Input: dimensioned drawing with shaded views. Units: mm. Origin: part minimum x, y, z. Round coordinates to 2 decimals unless told otherwise and drop trailing zeros. Loops run counter-clockwise (first coordinate to the right, second up) from the corner with the lowest first, then second, coordinate; pieces in that order, holes last. Notation, with made-up numbers: M -12,36 L -2,36 A24 ccw -2,72 Z; hole C 77,73.5 d5. An arc over 180 degrees is marked long. Answer as a JSON object with one key per item and string values.
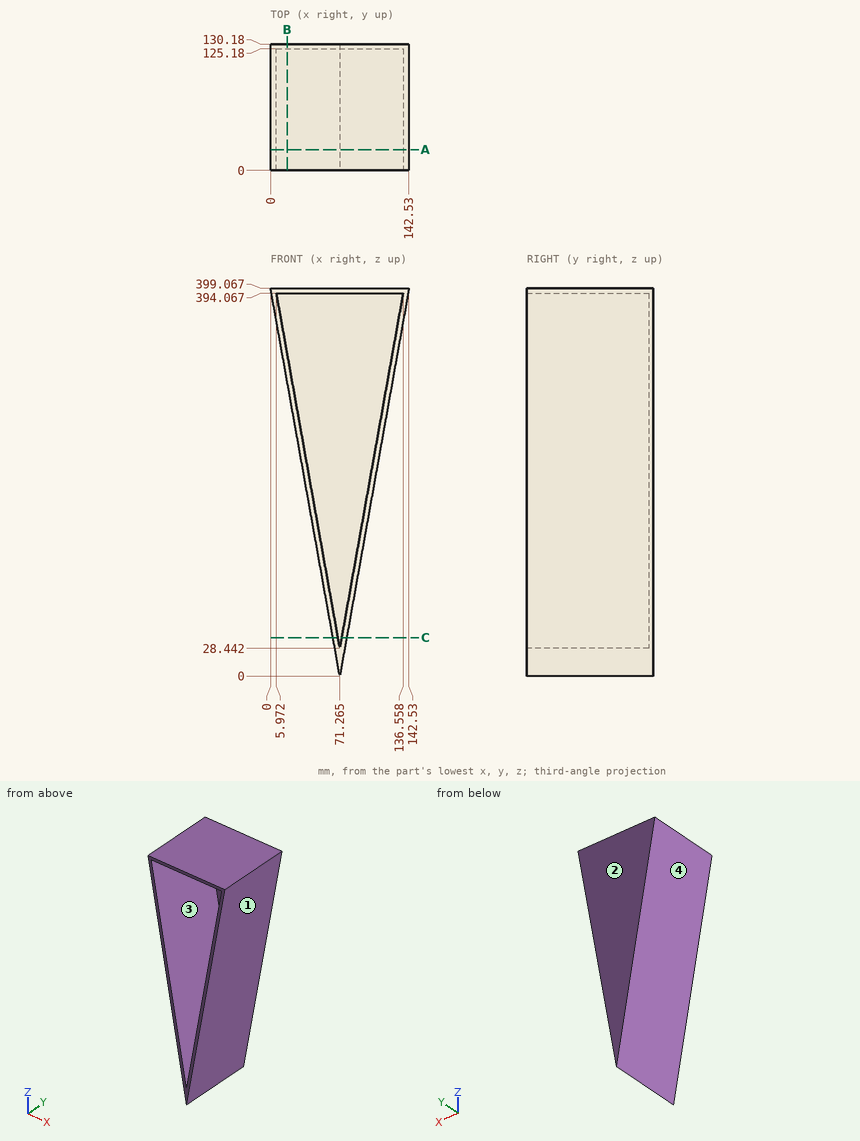
Item 1: Contact query for flat-ended pins moving along their axis: pin 1 Ø10 at (y, z) = (114, 351.5) entering from +X; pin 2 Ø8 at (x, z) = (59.5, 190.5) entering from -Y; pin 3 Ø2 at (y, z) = (90.5, 170.5) entering from -X. Output: stop coordinate, or through.
Answer sheet:
{"pin 1": "stops at x = 134.93", "pin 2": "stops at y = 125.18", "pin 3": "stops at x = 40.64"}
Item 2: Section A-A on y = 21.5. Return the cut outline in (x, z) (1 decimal), then the cut area to 3 significant figures.
Answer sheet:
{"outline": "M 0,399.1 L 71.3,0 L 142.5,399.1 Z; hole M 6,394.1 L 71.3,28.4 L 136.6,394.1 Z", "area": "4,570 mm²"}
Item 3: Section C-C on z = 39.5. Return the cut outline in (x, y).
Answer sheet:
{"outline": "M 64.21,0 L 69.29,0 L 69.29,125.18 L 73.24,125.18 L 73.24,0 L 78.32,0 L 78.32,130.18 L 64.21,130.18 Z"}
Item 4: Line query: probe 1 along X at (y, z) = (120, 265); probe 2 along Y at (x, z) = (74.5, 313.5); probe 3 along X at (y, z) = (87, 237). Output: solid intervals per line, ascending. Write a range as from..to.
Answer sheet:
{"probe 1": "x = 23.94..29.02, 113.51..118.59", "probe 2": "y = 125.18..130.18", "probe 3": "x = 28.94..34.02, 108.51..113.59"}
Item 5: Pull-direction query (X, two-part tool) for the marked faces 1, 2, 3 and 4; classes: pulls with the +X half, pulls with the -X half, needs draft (parallel to the pull), parting line crosses it, or undercut.
Answer sheet:
{"face 1": "pulls with the +X half", "face 2": "needs draft", "face 3": "undercut", "face 4": "pulls with the -X half"}
Item 6: Section B-B on x = 17. Return the cut outline in (y, z), then the cut area to 3 significant figures.
Answer sheet:
{"outline": "M 0,303.87 L 130.18,303.87 L 130.18,399.07 L 0,399.07 L 0,394.07 L 125.18,394.07 L 125.18,332.31 L 0,332.31 Z", "area": "4,660 mm²"}
